Read the model definition and answer for the solid it produces. Units are mm, in the model's axes. A direction names the side the tool comes from. Round coordinates to 2 decimals unless told otherwise and drop trailing zeros. Order: outer loops, then holes, each group sorted by start corner. A loop starts at its lowest first (then second) coordinate and runs counter-clockwise, first axis right, second up. Notation, with made-up numbers: (13, -4) - (71, -4) arc R15 cw to (71, 2) - close; hole circle Ø8 at (38, 19.5). An arc over 180 degrees is marked (long way). Put each result on its own line as item: value. Start each with the question number.
Q1. Section D-D on x = 2 is taken. Give the vertices of the cut face in (y, z), then the cut area to 3 significant figures.
Q2. Which of the six approach directions +Z, -Z, +X, -X, +Y, -Y give full straight-line access (tool end or side, diameter ignored) to faces 1 (the face through (15, 6, 1.08)), 2 (the face through (-7.36, 2.5, 0.02)), 3 (the face through (15.615, 0.833, 0.033)), 4 (the face through (-14.097, 4, -2))?
Q3. Section B-B on y = 5 is taken. Give the vertices of the cut face in (x, z), then the cut area to 3 significant figures.
Q4. For a pull along X with two mould halves and no side action, classify faces 5 (the face through (19.05, 4, 0)), 6 (the face through (18, 0, 0)), 7 (the face through (15, 5, -1.08)) as pulls with the +X half, pulls with the -X half, needs draft (parallel to the pull), parting line crosses it, or undercut.
Q5. Each of these flat-tipped pins is pushed along its axis until it touches: pin 1 Ø1.7 at (x, y) = (-1, 2.5) entering from -Z; pin 2 Ø3.5 at (x, y) = (6, 1.5) entering from +Z. Where does it stop, or does it pass through?
Q6. Find the intervals of material crossed by line 1 along Z through (x, y) = (-15.5, 4.25); line 2 along X through (y, z) = (0.75, 1.45); line 3 along X through (y, z) = (3, -1.5), in increasing order. Write a range as from..to.
from build123d import *

# Parameters (mm, degrees)
SKETCH1_W               = 38.1
SKETCH1_H               = 2.159
BOSS_EXTRUDE1_DEPTH     = 8.255
CUT_EXTRUDE1_DEPTH      = 12.7
SKETCH3_W               = 4.953
SKETCH3_H               = 8.255
BOSS_EXTRUDE2_DEPTH     = 1.27
FILLET5_R               = 0.4826
MIRROR2_COPY_1_SKETCH_W = 4.953
MIRROR2_COPY_1_SKETCH_H = 8.255
MIRROR2_COPY_1_DEPTH    = 1.27
CUT_EXTRUDE2_DEPTH      = 22.286806422
FILLET6_R               = 0.6985


with BuildPart() as part:
    # Sketch1 → Boss-Extrude1 (new body)
    with BuildSketch(Plane(origin=(0, 0, 0), x_dir=(1, 0, 0), z_dir=(0, 1, 0))):
        Rectangle(SKETCH1_W, SKETCH1_H)
    extrude(amount=BOSS_EXTRUDE1_DEPTH)

    # Sketch2 → Cut-Extrude1 (cut)
    with BuildSketch(Plane.XY.offset(1.0795)):
        with BuildLine():
            ThreePointArc((-0.435059279, 1.676786249), (0, 1.651), (0.435059279, 1.676786249))
            Line((0.435059279, 1.676786249), (14.097, 3.302))
            ThreePointArc((14.097, 3.302), (15.901602081, 5.334), (14.097, 7.366))
            Line((14.097, 7.366), (14.202754743, 8.255))
            Line((14.202754743, 8.255), (-14.202754743, 8.255))
            Line((-14.202754743, 8.255), (-14.097, 7.366))
            ThreePointArc((-14.097, 7.366), (-15.901602081, 5.334), (-14.097, 3.302))
            Line((-14.097, 3.302), (-0.435059279, 1.676786249))
        make_face()
    extrude(amount=-CUT_EXTRUDE1_DEPTH, mode=Mode.SUBTRACT)

    # Sketch3 → Boss-Extrude2 (add)
    with BuildSketch(Plane.XY.offset(1.0795)):
        with Locations((-16.5735, 4.1275)):
            Rectangle(SKETCH3_W, SKETCH3_H)
    boss_extrude2 = extrude(amount=BOSS_EXTRUDE2_DEPTH)

    # Fillet5
    fillet5_edges = [part.edges().sort_by_distance(p)[0] for p in [
        (14.202754743, 8.255, 0),
        (-14.202754743, 8.255, 0),
        (14.097, 7.366, 0),
        (-14.097, 7.366, 0),
    ]]
    fillet(fillet5_edges, radius=FILLET5_R)

    # Mirror1: Boss-Extrude2 across plane
    add(boss_extrude2.mirror(Plane(origin=(0, 0, 0), x_dir=(0, 0, 1), z_dir=(1, 0, 0))))

    # Mirror2: Boss-Extrude2 across plane
    add(boss_extrude2.mirror(Plane.XY))

    # Mirror2 copy 1 sketch → Mirror2 copy 1 (add)
    with BuildSketch(Plane(origin=(0, 0, -1.0795), x_dir=(-1, 0, 0), z_dir=(0, 0, -1))):
        with Locations((-16.5735, 4.1275)):
            Rectangle(MIRROR2_COPY_1_SKETCH_W, MIRROR2_COPY_1_SKETCH_H)
    extrude(amount=MIRROR2_COPY_1_DEPTH)

    # Sketch4 → Cut-Extrude2 (cut, through all)
    with BuildSketch(Plane.XY.offset(2.3495)):
        Polygon((15.3035, 1.6891), (17.8435, 1.6891), (17.228717877, 0), (15.918282123, 0), align=None)
    extrude(amount=-CUT_EXTRUDE2_DEPTH, mode=Mode.SUBTRACT)

    # Fillet6
    # the kernel refuses this fillet: 0.6985 mm, written as the material it takes off along each edge
    with BuildSketch(Plane(origin=(-19.05, 8.255, -4.09575), x_dir=(1, 0, 0), z_dir=(0, 0, 1)), Plane(origin=(19.05, 8.255, 4.09575), x_dir=(-1, 0, 0), z_dir=(0, 0, -1)), Plane(origin=(-19.05, 0, 4.09575), x_dir=(1, 0, 0), z_dir=(0, 0, -1))) as fillet6_piece_1:
        with BuildLine():
            CenterArc((FILLET6_R, -FILLET6_R), FILLET6_R, 90, 90)
            Line((0, -FILLET6_R), (0, 0))
            Line((0, 0), (FILLET6_R, 0))
        make_face()
    extrude(amount=8.1915, mode=Mode.SUBTRACT)
    with BuildSketch(Plane(origin=(-14.097, 8.255, 0.66675), x_dir=(-1, 0, 0), z_dir=(0, 0, -1)), Plane(origin=(-14.097, 8.255, -0.66675), x_dir=(0, -1, 0), z_dir=(0, 0, 1))) as fillet6_piece_2:
        with BuildLine():
            CenterArc((FILLET6_R, -FILLET6_R), FILLET6_R, 90, 90)
            Line((0, -FILLET6_R), (0, 0))
            Line((0, 0), (FILLET6_R, 0))
        make_face()
    extrude(amount=4.7625, mode=Mode.SUBTRACT)
    with BuildSketch(Plane(origin=(-14.097, 0, -1.0795), x_dir=(-1, 0, 0), z_dir=(0, 0, -1)), Plane(origin=(-14.097, 0, 1.0795), x_dir=(0, 1, 0), z_dir=(0, 0, 1))) as fillet6_piece_3:
        with BuildLine():
            CenterArc((FILLET6_R, FILLET6_R), FILLET6_R, 180, 90)
            Line((0, FILLET6_R), (0, 0))
            Line((0, 0), (FILLET6_R, 0))
        make_face()
    extrude(amount=3.01625, mode=Mode.SUBTRACT)
    with BuildSketch(Plane(origin=(14.097, 0, -1.0795), x_dir=(1, 0, 0), z_dir=(0, 0, -1)), Plane(origin=(14.097, 0, 1.0795), x_dir=(0, 1, 0), z_dir=(0, 0, 1))) as fillet6_piece_4:
        with BuildLine():
            CenterArc((FILLET6_R, -FILLET6_R), FILLET6_R, 90, 90)
            Line((0, -FILLET6_R), (0, 0))
            Line((0, 0), (FILLET6_R, 0))
        make_face()
    extrude(amount=3.01625, mode=Mode.SUBTRACT)
    with BuildSketch(Plane(origin=(14.097, 8.255, 0.66675), x_dir=(1, 0, 0), z_dir=(0, 0, -1)), Plane(origin=(14.097, 8.255, -0.66675), x_dir=(0, -1, 0), z_dir=(0, 0, 1))) as fillet6_piece_5:
        with BuildLine():
            CenterArc((FILLET6_R, FILLET6_R), FILLET6_R, 180, 90)
            Line((0, FILLET6_R), (0, 0))
            Line((0, 0), (FILLET6_R, 0))
        make_face()
    extrude(amount=4.7625, mode=Mode.SUBTRACT)
    with BuildSketch(Plane(origin=(19.05, 0, -4.09575), x_dir=(0, 1, 0), z_dir=(0, 0, 1))) as fillet6_piece_6:
        with BuildLine():
            CenterArc((FILLET6_R, FILLET6_R), FILLET6_R, 180, 90)
            Line((0, FILLET6_R), (0, 0))
            Line((0, 0), (FILLET6_R, 0))
        make_face()
    extrude(amount=8.1915, mode=Mode.SUBTRACT)


solid = part.part
Findings:
1. outline: (0, -1.08) - (1.86, -1.08) - (1.86, 1.08) - (0, 1.08) - close
1. area: 4.02 mm2
2. face 1: none
2. face 2: +Z, -Z, +Y
2. face 3: +Z, -Z
2. face 4: -Z, +Y, -Y
3. outline: (-19.05, -2.35) - (-14.1, -2.35) - (-14.1, -1.08) - (-15.87, -1.08) - (-15.87, 1.08) - (-14.1, 1.08) - (-14.1, 2.35) - (-19.05, 2.35) - close; (14.1, -2.35) - (19.05, -2.35) - (19.05, 2.35) - (14.1, 2.35) - (14.1, 1.08) - (15.87, 1.08) - (15.87, -1.08) - (14.1, -1.08) - close
3. area: 38.9 mm2
4. face 5: pulls with the +X half
4. face 6: needs draft
4. face 7: undercut
5. pin 1: z = -1.08
5. pin 2: z = 1.08
6. line 1: -2.35..-1.08, 1.08..2.35
6. line 2: -19.05..-14.1, 14.1..15.65, 17.5..19.05
6. line 3: -19.05..-14.1, 14.1..19.05
